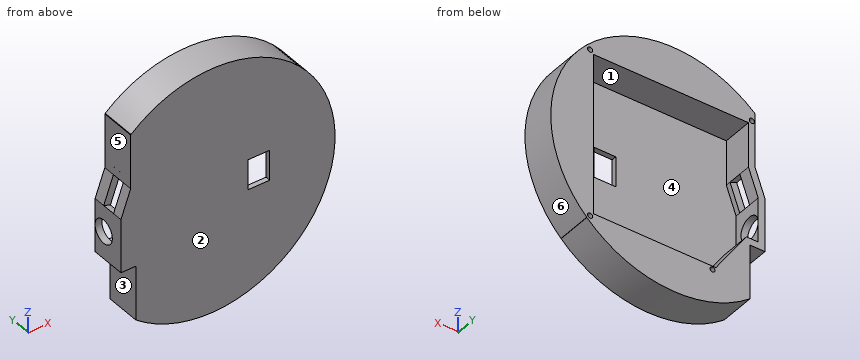
Autodesk Inventor part; units mm, degrees
ref_plane "YZ Plane" through (0, 0, 0) normal (1, 0, 0) x (0, 1, 0)
ref_plane "XZ Plane" through (0, 0, 0) normal (0, 1, 0) x (-1, 0, 0)
ref_plane "XY Plane" through (0, 0, 0) normal (0, 0, 1) x (1, 0, 0)
sketch "Sketch1" plane through (0, 0, 0) normal (0, 1, 0) x (-1, 0, 0)
  line L0 (0, 0) -> (49.1, 0)
  line L1 (49.1, -47.9) -> (0, -47.9)
  line L2 (0, -47.9) -> (0, 0)
  line L3 (46.7, -10.9) -> (49.1, -18.9)
  line L4 (46.7, -10.9) -> (46.7, 0)
  line L5 (49.1, 0) -> (46.7, 0)
  line L6 (49.1, -18.9) -> (49.1, -47.9)
  dimension "d0" = 49.1
  dimension "d1" = 47.9
  dimension "d2" = 18.9
extrude "Extrusion1" add sketch "Sketch1" along normal blind 1.5
sketch "Sketch2" plane through (0, 1.5, 0) normal (0, 1, 0) x (1, 0, 0)
  line L0 (-49.1, 18.9) -> (-46.7, 10.9)
  line L1 (-46.2, 10.9) -> (-46.2, 0)
  line L2 (-46.2, 0) -> (-46.7, 0)
  line L3 (-46.7, 10.9) -> (-46.7, 0)
  line L4 (-46.7, 0) -> (-46.7, 10.9)
  line L5 (-49.1, 47.9) -> (-49.1, 18.9)
  line L6 (-46.7, 10.9) -> (-49.1, 18.9)
  line L7 (-49.1, 18.9) -> (-46.2, 10.9)
  point P0 (0, 0)
extrude "Extrusion2" cut sketch "Sketch2" against normal blind 10
sketch "Sketch3" plane through (0, 1.5, 0) normal (0, 1, 0) x (1, 0, 0)
  line L0 (-49.1, 47.9) -> (-49.1, 18.9)
  line L1 (-49.1, 34.5784) -> (-45.5979, 34.5784)
  line L2 (-45.5979, 34.5784) -> (-36.4784, 47.9)
  line L3 (0, 47.9) -> (-49.1, 47.9)
  line L4 (-49.1, 47.9) -> (-36.4784, 47.9)
  line L5 (-49.1, 47.9) -> (-49.1, 34.5784)
  point P0 (0, 0)
extrude "Extrusion3" cut sketch "Sketch3" against normal blind 10
sketch "Sketch4" plane through (0, 1.5, 0) normal (0, 1, 0) x (1, 0, 0)
  line L0 (-46.2, 10.9) -> (-49.1, 18.9)
  line L1 (-46.2, 0) -> (0, 0)
  line L2 (-46.2, -2) -> (0, -2)
  line L3 (0, -2) -> (2, -2)
  line L4 (2, -2) -> (2, 47.9)
  line L5 (0, 47.9) -> (-36.4784, 47.9)
  line L6 (2, 47.9) -> (2, 49.9)
  line L7 (2, 49.9) -> (-36.4784, 49.9)
  line L8 (-38.1287, 49.0298) -> (-37.533, 49.9)
  line L9 (-37.533, 49.9) -> (-36.4784, 49.9)
  line L10 (-45.5979, 34.5784) -> (-36.4784, 47.9)
  line L11 (-49.1, 36.5784) -> (-46.6525, 36.5784)
  line L12 (-46.6525, 36.5784) -> (-37.533, 49.9)
  line L13 (-46.2, -2) -> (-48.2, -2)
  line L14 (-48.2, -2) -> (-48.2, 10.9)
  line L15 (-51.1, 18.9) -> (-48.2, 10.9)
  line L16 (-49.1, 36.5784) -> (-51.1, 36.5784)
  line L17 (-51.1, 36.5784) -> (-51.1, 18.9)
  line L18 (0, 0) -> (0, 47.9)
  line L19 (0, 0) -> (0, 47.9)
  line L20 (0, 47.9) -> (-36.4784, 47.9)
  line L21 (-36.4784, 47.9) -> (-45.5979, 34.5784)
  line L22 (-45.5979, 34.5784) -> (-49.1, 34.5784)
  line L23 (-49.1, 34.5784) -> (-45.5979, 34.5784)
  line L24 (-49.1, 34.5784) -> (-49.1, 18.9)
  line L25 (-49.1, 34.5784) -> (-49.1, 18.9)
  line L26 (-49.1, 18.9) -> (-46.2, 10.9)
  line L27 (-46.2, 0) -> (-46.2, 10.9)
  line L28 (-46.2, 0) -> (0, 0)
  dimension "d16" = 2
  dimension "d17" = 2
  dimension "d18" = 2
  dimension "d23" = 2
extrude "Extrusion4" add sketch "Sketch4" along normal blind 9
sketch "Sketch5" plane through (0, 0, 0) normal (0, -1, 0) x (1, 0, 0)
  line L0 (-46.2, 0) -> (0, 0)
  line L1 (0, 0) -> (-46.2, 0)
  line L2 (-46.2, 0) -> (-46.2, -10.9)
  line L3 (-46.2, 0) -> (-46.2, -10.9)
  line L4 (-46.2, -10.9) -> (-49.1, -18.9)
  line L5 (-46.2, -10.9) -> (-49.1, -18.9)
  line L6 (-49.1, -18.9) -> (-49.1, -34.5784)
  line L7 (-49.1, -18.9) -> (-49.1, -34.5784)
  line L8 (-49.1, -34.5784) -> (-45.5979, -34.5784)
  line L9 (-49.1, -34.5784) -> (-45.5979, -34.5784)
  line L10 (-36.4784, -47.9) -> (-45.5979, -34.5784)
  line L11 (-45.5979, -34.5784) -> (-36.4784, -47.9)
  line L12 (-36.4784, -47.9) -> (0, -47.9)
  line L13 (-36.4784, -47.9) -> (0, -47.9)
  line L14 (0, -47.9) -> (0, 0)
  line L15 (-48.2, 2) -> (2, 2)
  line L16 (2, 2) -> (-48.2, 2)
  line L17 (-51.1, -18.9) -> (-48.2, -10.9)
  line L18 (-48.2, 2) -> (-48.2, -10.9)
  line L19 (-48.2, -10.9) -> (-51.1, -18.9)
  line L20 (-51.1, -18.9) -> (-51.1, -36.5784)
  line L21 (-46.6525, -36.5784) -> (-51.1, -36.5784)
  line L22 (-51.1, -36.5784) -> (-46.6525, -36.5784)
  line L23 (-37.533, -49.9) -> (-46.6525, -36.5784)
  line L24 (-46.6525, -36.5784) -> (-37.533, -49.9)
  line L25 (2, 2) -> (2, -49.9)
  line L26 (-37.533, -49.9) -> (2, -49.9)
  line L27 (2, -49.9) -> (2, 2)
extrude "Extrusion5" add sketch "Sketch5" against normal blind 1.5
sketch "Sketch6" plane through (0, 10.5, 0) normal (0, 1, 0) x (1, 0, 0)
  line L0 (-48.2, -2) -> (2, -2)
  circle A0 centre (1, -1) radius 0.75
  line L1 (-46.2, 0) -> (-46.2, 10.9)
  circle A1 centre (-47.2, -1) radius 0.75
  point P0 (0, 0)
  dimension "d35" = 1.5
sketch "Sketch7" plane through (0, 10.5, 0) normal (0, 1, 0) x (1, 0, 0)
  point P0 (0, 0)
extrude "Extrusion6" cut sketch "Sketch6" against normal blind 7.5
sketch "Sketch8" plane through (0, 10.5, 0) normal (0, 1, 0) x (1, 0, 0)
  line L0 (-45.5979, 34.5784) -> (-36.4784, 47.9)
  circle A0 centre (-35.4784, 48.9) radius 0.75
  circle A1 centre (1, 48.9) radius 0.75
  point P0 (0, 0)
  dimension "d40" = 1.5
  dimension "d43" = 1.5
extrude "Extrusion7" cut sketch "Sketch8" against normal blind 7.5
sketch "Sketch9" plane through (0, 0, 0) normal (0, -1, 0) x (1, 0, 0)
  line L0 (-48.2, 2) -> (2, 2)
  line L1 (2, 2) -> (2, -49.9)
  line L2 (-6.75, -23.95) -> (-6.75, -19.45)
  line L3 (-6.75, -19.45) -> (-13.25, -19.45)
  line L4 (-13.25, -19.45) -> (-13.25, -28.45)
  line L5 (-13.25, -28.45) -> (-6.75, -28.45)
  line L6 (-6.75, -28.45) -> (-6.75, -23.95)
  point P0 (0, 0)
  dimension "d51" = 6.5
  dimension "d52" = 9
extrude "Extrusion8" cut sketch "Sketch9" against normal blind 1.5
sketch "Sketch10" plane through (0, 10.5, 0) normal (0, 1, 0) x (1, 0, 0)
  line L0 (-49.1, 18.9) -> (-46.2, 10.9)
  line L1 (-48.2, -2) -> (-48.2, 10.9)
  line L2 (-48.2, 10.9) -> (-51.1, 18.9)
  line L3 (-48.2, 10.175) -> (-48.2, 10.9)
  line L4 (-51.1, 18.9) -> (-51.1, 36.5784)
  line L5 (-51.1, 18.175) -> (-51.1, 18.9)
  line L6 (-51.1, 18.175) -> (-48.2, 10.175)
  line L7 (-48.2, 10.9) -> (-51.1, 18.9)
  point P0 (0, 0)
extrude "Extrusion9" add sketch "Sketch10" against normal blind 10.5
sketch "Sketch11" plane through (-51.1, 0, -18.175) normal (-0.9401361, 0, 0.3407993) x (0.3407993, 0, 0.9401361)
  point P0 (34.5018, 0)
sketch "Sketch12" plane through (-51.1, 0, -18.175) normal (-0.9401361, 0, 0.3407993) x (0.3407993, 0, 0.9401361)
  line L0 (0, 10.5) -> (0, 0)
  line L1 (5.4546, 0) -> (3.2394, 0)
  line L2 (4.2545, 0) -> (7.2545, 0) construction
  line L3 (4.2545, 7) -> (0, 7)
  line L4 (0, 7) -> (0, 3)
  line L5 (0, 3) -> (8.5094, 3)
  line L6 (8.5094, 1.5) -> (8.5094, 10.5)
  line L7 (4.2545, 7) -> (8.5094, 7)
  line L8 (8.5094, 10.5) -> (8.5094, 0)
  line L9 (8.5094, 3) -> (8.5094, 7)
  line L10 (0, 10.5) -> (8.5094, 10.5)
  line L11 (0, 10.5) -> (0, 0)
  line L12 (8.5094, 0) -> (0, 0)
  line L13 (8.5094, 10.5) -> (8.5094, 0)
  point P0 (34.5018, 0)
  dimension "d58" = 4.2545
extrude "Extrusion10" cut sketch "Sketch12" along normal blind 5 contours L3 L7 L6 L5 L0
sketch "Sketch14" plane through (0, 10.5, 0) normal (0, 1, 0) x (1, 0, 0)
  point P0 (0, 0)
sketch "Sketch15" plane through (0, 10.5, 0) normal (0, 1, 0) x (1, 0, 0)
  line L0 (-46.2, 0) -> (-46.2, 10.9)
  line L1 (-46.2, 10.9) -> (-46.2, 11.9)
  line L2 (-46.2, 11.9) -> (-49.1, 19.8981)
  line L3 (-49.1, 34.5784) -> (-49.1, 18.9)
  line L4 (-46.2, 11.9) -> (-37.6924, 11.9) construction
  line L5 (-49.1, 19.8981) -> (-49.1, 18.9)
  line L6 (-49.1, 18.9) -> (-46.2, 10.9)
  line L7 (-49.1, 18.9) -> (-46.2, 10.9)
  point P0 (0, 0)
  dimension "d71" = 1
  dimension "d72" = 109.93
extrude "Extrusion12" add sketch "Sketch15" against normal blind 9
sketch "Sketch16" plane through (0, 10.5, 0) normal (0, 1, 0) x (1, 0, 0)
  line L0 (-51.1, 18.175) -> (-48.2, 10.175)
  line L1 (-51.1, 18.175) -> (-51.1, 19.175)
  line L2 (-51.1, 36.5784) -> (-51.1, 18.175)
  line L3 (-51.1, 19.175) -> (-48.2, 11.1769)
  line L4 (-51.1, 19.175) -> (-42.5924, 19.175) construction
  line L5 (-48.2, 11.1769) -> (-48.2, 10.175)
  line L6 (-48.2, 10.175) -> (-48.2, -2)
  line L7 (-51.1, 18.175) -> (-48.2, 10.175)
  point P0 (0, 0)
  dimension "d75" = 1
  dimension "d76" = 70.07
extrude "Extrusion13" cut sketch "Sketch16" against normal blind 10.5
sketch "Sketch17" plane through (-51.1, 0, -36.5784) normal (-1, 0, 0) x (0, 0, 1)
  line L0 (-13.3216, 0) -> (-13.3216, 10.5)
  line L1 (36.8284, 10.5) -> (36.8284, 3)
  line L2 (38.5784, 0) -> (38.5784, 10.5)
  line L3 (15.9784, 5.25) -> (15.9784, 10.5) construction
  line L4 (16.6804, 10.5) -> (2, 10.5)
  point P0 (36.5784, 0)
sketch "Sketch18" plane through (0, 10.5, 0) normal (0, 1, 0) x (1, 0, 0)
  line L0 (-51.1, 19.175) -> (-51.1, 36.5784)
  line L1 (-51.1, 19.175) -> (-51.1, 20.6)
  line L2 (-51.1, 20.6) -> (-48.2, 12.6019)
  line L3 (-51.1, 20.6) -> (-42.5924, 20.6) construction
  line L4 (-51.1, 19.175) -> (-48.2, 11.1769)
  line L5 (-48.2, 12.6019) -> (-48.2, 11.1769)
  line L6 (-51.1, 19.175) -> (-48.2, 11.1769)
  point P0 (0, 0)
  dimension "d82" = 1.425
  dimension "d83" = 70.07
extrude "Extrusion14" cut sketch "Sketch18" against normal blind 10.5
sketch "Sketch19" plane through (0, 10.5, 0) normal (0, 1, 0) x (1, 0, 0)
  line L0 (-46.2, 11.9) -> (-49.1, 19.8981)
  line L1 (-46.2, 11.9) -> (-46.2, 13.325)
  line L2 (-46.2, 13.325) -> (-49.1, 21.3231)
  line L3 (-49.1, 19.8981) -> (-49.1, 34.5784)
  line L4 (-49.1, 21.3231) -> (-49.1, 19.8981)
  line L5 (-49.1, 19.8981) -> (-46.2, 11.9)
  point P0 (0, 0)
  dimension "d86" = 1.425
  dimension "d87" = 160.07
extrude "Extrusion15" add sketch "Sketch19" against normal blind 9
sketch "Sketch20" plane through (-51.1, 0, -20.6) normal (-0.9401098, 0, 0.3408718) x (0.3408718, 0, 0.9401098)
  line L0 (0, 3) -> (8.5096, 3)
  line L1 (8.5096, 10.5) -> (8.5096, 1.5)
  line L2 (8.5096, 3) -> (8.5096, 7)
  line L3 (8.5096, 7) -> (0.002, 7)
  line L4 (0.002, 10.5) -> (0.002, 1.5)
  line L5 (0, 3) -> (0.002, 7)
  point P0 (36.7848, 0)
  point P1 (0, 0)
  point P2 (8.5096, 7)
  dimension "d90" = 3
  dimension "d91" = 4
extrude "Extrusion16" cut sketch "Sketch20" against normal blind 10
sketch "Sketch21" plane through (-51.1, 0, -36.5784) normal (-1, 0, 0) x (0, 0, 1)
  point P0 (36.5784, 0)
sketch "Sketch22" plane through (-51.1, 0, -36.5784) normal (-1, 0, 0) x (0, 0, 1)
  line L0 (15.9784, 0) -> (0, 0)
  line L1 (17.1284, 0) -> (8.1284, 0)
  circle A0 centre (8.1284, 7) radius 3.5
  point P0 (36.5784, 0)
  dimension "d98" = 7
extrude "Extrusion17" cut sketch "Sketch22" against normal blind 10
sketch "Sketch23" plane through (0, 10.5, 0) normal (0, 1, 0) x (1, 0, 0)
  line L0 (2, -2) -> (2, 49.9)
  line L1 (2, 23.95) -> (-23.95, 23.95)
  arc A0 (-48.065, -3.674) -> (-46.6525, 52.746) centre (-23.95, 23.95) ccw
  line L2 (2, -2) -> (-48.2, -2)
  line L3 (-48.2, -2) -> (-48.2, -3.5555)
  line L4 (-48.2, -3.5555) -> (-48.065, -3.674)
  line L5 (-46.6525, 36.5784) -> (-46.6525, 52.746)
  line L6 (-48.2, -2) -> (2, -2)
  line L7 (2, -2) -> (2, 49.9)
  line L8 (2, 49.9) -> (-37.533, 49.9)
  line L9 (-37.533, 49.9) -> (-46.6525, 36.5784)
  point P0 (0, 0)
  point P1 (1.9578, 49.9)
  point P2 (2, -1.9578)
  point P3 (2, 49.8578)
  point P4 (1.9578, -2)
  dimension "d114" = 25.95
  dimension "d115" = 36.669
extrude "Extrusion18" add sketch "Sketch23" against normal blind 10.5 contours A0 L4 L3 L2 | L8 L9 L5 A0 | L0 A0
properties part number "Case"
Geometry check sheet. Reference: the model listing, model coordinates, mm. Face numbers are marked on the shaded views. A direction names the side the tool comes from. Round coordinates to 2 decimals unless told otherwise and drop trailing zeros. Loops run counter-clockwise (first coordinate to the right, second up) from the corner with the lowest first, then second, coordinate; pieces in that order, holes last. Notation, with made-up numbers: (75, 56.25) - (97, 56.25) arc R30 cw to (97, 83.25) - close; hole circle Ø3 at (20.25, 51.25). An arc over 180 degrees is marked (long way). Use a Markdown table: item, result.
Q1. Cross-section at A-A on y = 5. State how many separate pieces and enclosed holes the cut face has, plus the area to 3 significant figures.
Solutions:
| item | result |
|---|---|
| separate pieces | 2 |
| enclosed holes | 4 |
| area | 1,550 mm2 |
Q2. Cross-section at C-C on x = -10.5. Record the cut outline in (y, z), plus the area to 3 significant figures.
Solutions:
| item | result |
|---|---|
| outline | (0, -58.06) - (10.5, -58.06) - (10.5, -47.9) - (1.5, -47.9) - (1.5, -28.45) - (0, -28.45) - close; (0, -19.45) - (1.5, -19.45) - (1.5, 0) - (10.5, 0) - (10.5, 10.16) - (0, 10.16) - close |
| area | 272 mm2 |
Q3. Material ranges on line 1 (Z direction, x = 1, y = 6.75); line 2 (X direction, y = 10.25, z = -24); line 3 (Y direction, x = -12.5, z = -33.5), recorded low to high.
Solutions:
| item | result |
|---|---|
| line 1 | z = -50.82 to -49.65, -48.15 to 0.25, 1.75 to 2.92 |
| line 2 | x = -51.1 to -49.1, 0 to 12.72 |
| line 3 | y = 0 to 1.5 |
Q4. Access from +Z, -Z, +X, -X, +Y, -Y to the whole of each face (thin tool, end or side, straight path). Record for the marked faces 1, 2 and 3.
Solutions:
| item | result |
|---|---|
| face 1 | +Y |
| face 2 | +Z, -Z, +X, -X, -Y |
| face 3 | -Z, -X, +Y, -Y |
Q5. Draft check along Z on the marked faces 4, 5 and 6. Enter one of: released by +Z, released by -Z, zero draft, split by the parting line, or undercut.
Solutions:
| item | result |
|---|---|
| face 4 | undercut |
| face 5 | zero draft |
| face 6 | split by the parting line |
Q6. Cross-section at D-D on x = -29. Record the cut outline in (y, z).
Solutions:
| item | result |
|---|---|
| outline | (0, -60.27) - (10.5, -60.27) - (10.5, -47.9) - (1.5, -47.9) - (1.5, 0) - (10.5, 0) - (10.5, 12.37) - (0, 12.37) - close |
Q7. Cross-section at B-B on z = -23. Record the cut outline in (x, y).
Solutions:
| item | result |
|---|---|
| outline | (-51.1, 0) - (-13.25, 0) - (-13.25, 1.5) - (-49.1, 1.5) - (-49.1, 10.5) - (-51.1, 10.5) - close; (-6.75, 0) - (12.71, 0) - (12.71, 10.5) - (0, 10.5) - (0, 1.5) - (-6.75, 1.5) - close |
Q8. Go/stop test with flat-tipped pins: P1, Ø1.4, axis at x = -47.2, z = 1, coming from the +Y side; P2, Ø5, axis at x = -24, y = 1.5, coming from the +Z side; P3, Ø2, axis at x = -48, y = 7, coming from the -Z side. Record where each tip stops, or that it passes through.
Solutions:
| item | result |
|---|---|
| P1 | stops at y = 3 |
| P2 | stops at z = 12.72 |
| P3 | stops at z = -36.58 |
